Verification items for the finished model (mm, model axes). A direction names the side the tool comes from. Give positions to 0.01 mm unless a question says otherwise; leave off trailing zeros. Order: outer loops, then holes, each group sorted by start corner. A loop starts at its lowest first (then second) coordinate and runs counter-clockwise, first axis right, second up. Notation, with made-up numbers: (-23, 46) - (-4, 46) arc R26 cw to (-4, 66) - close; hole circle Ø9 at (38.5, 57). An arc over 180 degrees is marked (long way). Answer as a JSON object with one key per item and string values. Group by question number.
(1) Depth check by flat-ended pin: pin 1 Ø2 at (y, z) = (5.5, -7.5) entering from -X; pin 2 Ø6 at (x, z) = (3, 7) entering from -Y; pin 3 Ø4 at (x, y) = (9.5, -5) entering from -Z; pin 4 Ø1.5 at (x, y) = (-2.5, 0.5) entering from +Z (3 decimals). Enter the tip coordinate at first touch or a pass-through.
(2) Access from +Z, -Z, +X, -X, +Y, -Y to the whole of each face (thin tool, end or side, straight path). Record for faces 5 (the face through (0.166, 4.643, -8.194)), 6 (the face through (-6.8, -1, -7)), 7 (the face through (6.8, 0, -7)).
(3) Thickness scan on line 1 (Y direction, x = 3.75, z = -0.25); line 2 (X direction, y = 8, z = -3.5); line 3 (Z direction, x = 6, y = -3). Record the ranges inside material, lowest first.
(4) Section check A-A (z = 0). Record the boundary of the cut face in (x, y) (3 decimals).
(5) Mould release check, pull along Z, two halves, no side actions. Record for faces 1 (the face through (0, 9.418, 0)), 2 (the face through (-10.02, -1.38, -6.2)), 3 (the face through (-0.32, -1.08, -4.88)), 4 (the face through (0.17, 4.77, 8.12)): +Z half, -Z half, draft (parallel to the pull), parting line (faces both ways), or undercut.
(6) Section check B-B (x = 3). Record the boundary of the cut face in (y, z) (1 decimal).
```python
from build123d import *

# Parameters (mm, degrees)
F0_R          = 6.35
F1_DEPTH      = 6.8
F1_DEPTH_BACK = 6.8
F2_DEPTH      = 13.82
F2_DEPTH_BACK = 12.8
F5_R          = 5
F6_DEPTH      = 15
F7_SIZE2      = 0.5773502692
F7_SIZE       = 1
F8_SIZE       = 0.5
F9_R          = 0.5


with BuildPart() as f1:
    # F0 (on Right) → F1 (new body, two sides)
    with BuildSketch(Plane.YZ) as f1_sk:
        Polygon((9.4180262662, 5.4375), (0, 10.875), (-9.4180262662, 5.4375), (-9.4180262662, -5.4375), (0, -10.875), (9.4180262662, -5.4375), align=None)
        Circle(F0_R, mode=Mode.SUBTRACT)
        Circle(F0_R)
    extrude(amount=F1_DEPTH)
    extrude(f1_sk.sketch, amount=-F1_DEPTH_BACK)

    # F0 (on Right) → F2 (join, two sides)
    with BuildSketch(Plane.YZ) as f2_sk:
        Circle(F0_R)
    extrude(amount=-F2_DEPTH)
    extrude(f2_sk.sketch, amount=F2_DEPTH_BACK)

    # F3 (on Front) → F4 (revolve, cut)
    with BuildSketch(Plane.XZ):
        Polygon((-6.8, 9.275), (-5.2, 10.875), (-6.8, 10.875), align=None)
    revolve(axis=Axis((0, 0, 0), (1, 0, 0)), mode=Mode.SUBTRACT)

    # F5 (on Right) → F6 (cut, symmetric)
    with BuildSketch(Plane.YZ):
        Circle(F5_R)
    extrude(amount=F6_DEPTH, both=True, mode=Mode.SUBTRACT)

    # F7
    f7_edges = [f1.edges().sort_by_distance(p)[0] for p in [
        (-13.82, -6.35, 0),
    ]]
    f7_side = f1.faces().sort_by_distance((-10.31, -6.35, 0))[0]
    chamfer(f7_edges, length=F7_SIZE, length2=F7_SIZE2, reference=f7_side)

    # F8
    f8_edges = [f1.edges().sort_by_distance(p)[0] for p in [
        (12.8, -6.35, 0),
    ]]
    chamfer(f8_edges, length=F8_SIZE)

    # F9
    f9_edges = [f1.edges().sort_by_distance(p)[0] for p in [
        (6.8, -6.35, 0),
        (-6.8, -6.35, 0),
    ]]
    fillet(f9_edges, radius=F9_R)


solid = f1.part
```
Solutions:
{
 "1": {"pin 1": "stops at x = -6.8", "pin 2": "stops at y = -9.42", "pin 3": "stops at z = -5.6", "pin 4": "stops at z = 10.875"},
 "2": {"face 5": "-Z, +X, -X, +Y", "face 6": "-X", "face 7": "+X"},
 "3": {"line 1": "y = -9.42 to -4.99, 4.99 to 9.42", "line 2": "x = -6.8 to 6.8", "line 3": "z = -9.14 to -4, 4 to 9.14"},
 "4": {"outline": "(-13.82, -5.773) - (-12.82, -6.35) - (-7.3, -6.35) arc R0.5 cw to (-6.8, -6.85) - (-6.8, -9.275) - (-6.657, -9.418) - (6.8, -9.418) - (6.8, -6.85) arc R0.5 cw to (7.3, -6.35) - (12.3, -6.35) - (12.8, -5.85) - (12.8, -5) - (-13.82, -5) - close; (-13.82, 5) - (12.8, 5) - (12.8, 5.85) - (12.3, 6.35) - (7.3, 6.35) arc R0.5 cw to (6.8, 6.85) - (6.8, 9.418) - (-6.657, 9.418) - (-6.8, 9.275) - (-6.8, 6.85) arc R0.5 cw to (-7.3, 6.35) - (-12.82, 6.35) - (-13.82, 5.773) - close"},
 "5": {"face 1": "draft", "face 2": "parting line", "face 3": "undercut", "face 4": "+Z half"},
 "6": {"outline": "(-9.4, -5.4) - (0, -10.9) - (9.4, -5.4) - (9.4, 5.4) - (0, 10.9) - (-9.4, 5.4) - close; hole circle Ø10 at (0, 0)"}
}
